Check sheet for the drawn part. Datum: minimum x, y, z corner. Units: mm. A direction names the side the tool comes from. Round coordinates to 2 decimals unless told otherwise and drop trailing zeros. Write each loop counter-clockwise with the first axis right and the second up, starting at its lowest first coordinate (ties: lowest second). Pieces come first, ordered by that corner, then holes. Notation, with made-up numbers: (52.5, -21.5) -> (107.5, -21.5) arc R27 ccw to (107.5, 10.5) -> close; hole circle Ø7 at (61, 9.5). An arc over 180 degrees is marked (long way). One line per item, written item: value.
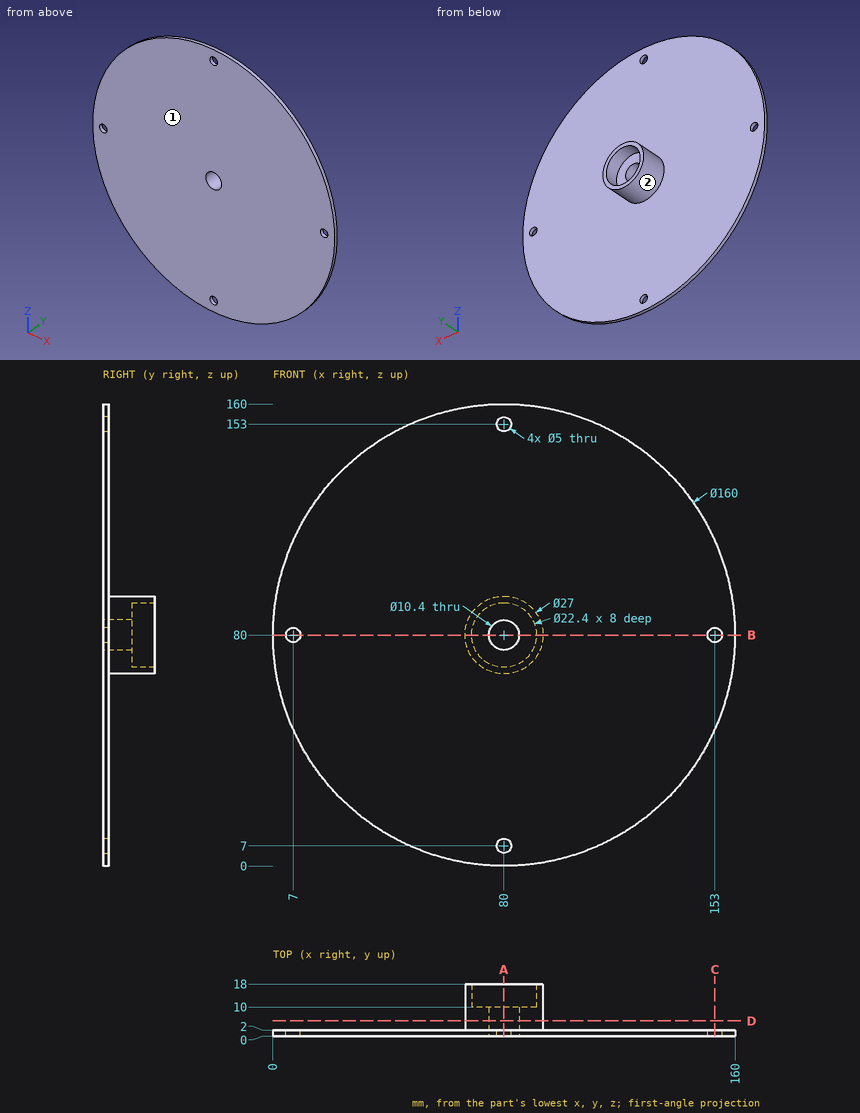
Item 1: Sectioned sample at C-C on x = 153. Enter the section's corners in (y, z).
Answer:
outline: (0, 47.27) -> (2, 47.27) -> (2, 77.5) -> (0, 77.5) -> close; (0, 82.5) -> (2, 82.5) -> (2, 112.73) -> (0, 112.73) -> close
Item 2: Sectioned sample at A-A on x = 80. Enter the section's corners in (y, z), and give its area (3 significant figures).
Answer:
outline: (0, 0) -> (2, 0) -> (2, 4.5) -> (0, 4.5) -> close; (0, 9.5) -> (2, 9.5) -> (2, 66.5) -> (18, 66.5) -> (18, 68.8) -> (10, 68.8) -> (10, 74.8) -> (0, 74.8) -> close; (0, 85.2) -> (10, 85.2) -> (10, 91.2) -> (18, 91.2) -> (18, 93.5) -> (2, 93.5) -> (2, 150.5) -> (0, 150.5) -> close; (0, 155.5) -> (2, 155.5) -> (2, 160) -> (0, 160) -> close
area: 449 mm^2
Item 3: Depth check by flat-ended pin: P1, Ø4.5, axis at x = 80, z = 7, coming from the +Y side; P2, Ø3, axis at y = 4.5, z = 91, coming from the +X side; P3, Ø8, axis at x = 90.5, y = 7, coming from the +Z side; P4, Ø4, axis at x = 100, z = 59.5, coming from the +Y side. Enter the tip coordinate at first touch or a pass-through.
Answer:
P1: passes through
P2: stops at x = 89.59
P3: stops at z = 91.83
P4: stops at y = 2
Item 4: Sectioned sample at B-B on z = 80. Enter the section's corners in (x, y), and give its area (3 significant figures).
Answer:
outline: (0, 0) -> (4.5, 0) -> (4.5, 2) -> (0, 2) -> close; (9.5, 0) -> (74.8, 0) -> (74.8, 10) -> (68.8, 10) -> (68.8, 18) -> (66.5, 18) -> (66.5, 2) -> (9.5, 2) -> close; (85.2, 0) -> (150.5, 0) -> (150.5, 2) -> (93.5, 2) -> (93.5, 18) -> (91.2, 18) -> (91.2, 10) -> (85.2, 10) -> close; (155.5, 0) -> (160, 0) -> (160, 2) -> (155.5, 2) -> close
area: 449 mm^2
Item 5: Tool access check on the marked faces 1 and 2. Record the directions out of +Z, -Z, +X, -X, +Y, -Y that give a thin tool (end or side, any length) a straight path to the whole face; none if there is none.
Answer:
face 1: +Z, -Z, +X, -X, -Y
face 2: +Y
Item 6: Sectioned sample at D-D on y = 5.25. Enter the section's corners in (x, z), and give its area (3 significant figures).
Answer:
outline: circle Ø27 at (80, 80); hole circle Ø10.4 at (80, 80)
area: 488 mm^2
Item 7: Thickness scan on line 1 (X direction, y = 14.5, z = 80); line 2 (Y direction, x = 85, z = 150); line 3 (X direction, y = 0.65, z = 7). Record the ranges inside material, lowest first.
Answer:
line 1: x = 66.5 to 68.8, 91.2 to 93.5
line 2: y = 0 to 2
line 3: x = 47.27 to 77.5, 82.5 to 112.73
